```python
from build123d import *

# Parameters (mm, degrees)
BOSS_EXTRUDE1_DEPTH = 250
CUT_EXTRUDE1_DEPTH  = 150


with BuildPart() as part:
    # Sketch1 → Boss-Extrude1 (new body)
    with BuildSketch(Plane.XY):
        Polygon((0, 0), (0, 22), (2, 22), (2, 2), (17, 2), (17, 0), align=None)
    extrude(amount=BOSS_EXTRUDE1_DEPTH)

    # Sketch2 → Cut-Extrude1 (cut)
    with BuildSketch(Plane(origin=(17, 0, 0), x_dir=(0, 0, -1), z_dir=(1, 0, 0))):
        Polygon((-216.454364826, 22), (-250, 22), (-250, 0), (-194.454364826, 0), align=None)
        Polygon((-22, 22), (0, 22), (0, 0), align=None)
    extrude(amount=-CUT_EXTRUDE1_DEPTH, mode=Mode.SUBTRACT)


solid = part.part
```
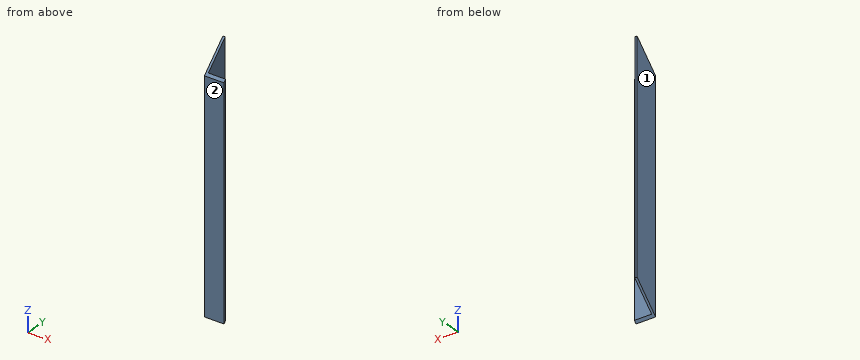
The listing builds one solid part. Answer for the finished solid, in the listing's coordinates (mm). Face numbers are marked on the shaded views. Coordinates: 2 decimals unless noted, no trailing zeros. Loops run counter-clockwise (first coordinate to the right, second up) from the corner with the lowest first, then second, coordinate; pieces in that order, holes last. Notation, with made-up numbers: M 32,87.5 L 81,87.5 A20 cw 81,91.5 Z; hole C -30,-4.75 d1. An arc over 180 degrees is marked long. Answer as CSV lines item,"result". Start each with the question number.
(1) Given pin 1 (3 mm diameter, centred on y = 7, z = 176, fed in from +X); pin 2 (10 mm diameter, centred on x = 14, z = 23, fed in from +Y), each flat-ended and moving along its own axis, determine where each tip first touches the part or whether it passes through.
(2) Find the intervals of material crossed by L1, parallel to Y at x = 5.75, z = 72; L2, parallel to Z at x = 1, y = 8.5, in increasing order. Write a range as [from, to].
(3) The part is cut by section D-D (z = 154). Give the vertices of the cut face in (x, y).
(4) The mould has two halves that part along Y. Classify the marked faces 1 and 2: pulls with the +Y half, pulls with the -Y half, needs draft (parallel to the pull), parting line crosses it, or undercut.
(5) The part is cut by section C-C (y = 14.5). Give the vertices of the cut face in (x, z).
(6) The part is cut by section B-B (x = 11.5). Give the vertices of the cut face in (y, z), and give its area (3 significant figures).
(7) The part is cut by section A-A (z = 15.5). Give the vertices of the cut face in (x, y).
Determined:
1,pin 1,"x = 2"
1,pin 2,"y = 2"
2,L1,"[0, 2]"
2,L2,"[8.5, 202.95]"
3,outline,"M 0,0 L 17,0 L 17,2 L 2,2 L 2,22 L 0,22 Z"
4,face 1,"needs draft"
4,face 2,"pulls with the -Y half"
5,outline,"M 0,14.5 L 2,14.5 L 2,208.95 L 0,208.95 Z"
6,outline,"M 0,0 L 2,2 L 2,196.45 L 0,194.45 Z"
6,area,"389 mm2"
7,outline,"M 0,0 L 17,0 L 17,2 L 2,2 L 2,15.5 L 0,15.5 Z"
